The model under review builds one solid part; all positions refer to its coordinate system, in mm. A direction names the side the tool comes from. Coordinates: 2 decimals unless noted, no trailing zeros. Order: outer loops, then holes, each group sorted by start corner. A loop starts at its lowest first (then second) coordinate and runs counter-clockwise, first axis right, second up.
```python
from build123d import *

# Parameters (mm, degrees)
CROQUIS1_W              = 46
CROQUIS1_H              = 101
SALIENTE_EXTRUIR2_DEPTH = 4
CROQUIS2_R              = 2
CORTAR_EXTRUIR3_DEPTH   = 36
CROQUIS4_R              = 3
CORTAR_EXTRUIR4_DEPTH   = 2
REDONDEO1_R             = 5


with BuildPart() as part:
    # Croquis1 → Saliente-Extruir2 (new body)
    with BuildSketch(Plane(origin=(0, 0, 0), x_dir=(1, 0, 0), z_dir=(0, 1, 0))):
        Rectangle(CROQUIS1_W, CROQUIS1_H)
    extrude(amount=SALIENTE_EXTRUIR2_DEPTH)

    # Croquis2 → Cortar-Extruir3 (cut)
    with BuildSketch(Plane(origin=(0, 4, 0), x_dir=(1, 0, 0), z_dir=(0, 1, 0))):
        with Locations(Location((-15, 38.5, 0), (0, 0, 270))):
            Circle(CROQUIS2_R)
        with Locations(Location((15, 38.5, 0), (0, 0, 270))):
            Circle(CROQUIS2_R)
        with Locations(Location((-15, -38.5, 0), (0, 0, 270))):
            Circle(CROQUIS2_R)
        with Locations(Location((15, -38.5, 0), (0, 0, 270))):
            Circle(CROQUIS2_R)
    extrude(amount=-CORTAR_EXTRUIR3_DEPTH, mode=Mode.SUBTRACT)

    # Croquis4 → Cortar-Extruir4 (cut)
    with BuildSketch(Plane(origin=(0, 4, 0), x_dir=(1, 0, 0), z_dir=(0, 1, 0))):
        with Locations(Location((-15, -38.5, 0), (0, 0, 270))):
            Circle(CROQUIS4_R)
        with Locations(Location((15, -38.5, 0), (0, 0, 270))):
            Circle(CROQUIS4_R)
        with Locations(Location((-15, 38.5, 0), (0, 0, 270))):
            Circle(CROQUIS4_R)
        with Locations(Location((15, 38.5, 0), (0, 0, 270))):
            Circle(CROQUIS4_R)
    extrude(amount=-CORTAR_EXTRUIR4_DEPTH, mode=Mode.SUBTRACT)

    # Redondeo1
    redondeo1_edges = [part.edges().sort_by_distance(p)[0] for p in [
        (23, 2, 50.5),
        (-23, 2, 50.5),
        (-23, 2, -50.5),
        (23, 2, -50.5),
    ]]
    fillet(redondeo1_edges, radius=REDONDEO1_R)


solid = part.part
```
(1) Wall thickness on probe 1 along X at (y, z) = (1.2, -38.5); probe 2 along X at (y, z) = (3.55, -38.5); probe 3 along Z at (x, y) = (15.5, 1.4): over which ranges is each line inside the solid? List them lowest first.
A:
probe 1: x = -23 to -17, -13 to 13, 17 to 23
probe 2: x = -23 to -18, -12 to 12, 18 to 23
probe 3: z = -50.5 to -40.44, -36.56 to 36.56, 40.44 to 50.5
(2) Draft analysis for pull direction Z (two halves, no side actions). For faces 3 (the face through (0, 2, -50.5)), 4 (the face through (15, 2, 36)), 5 (the face through (0, 4, -1)), state which applies: released by +Z, released by -Z, zero draft, split by the parting line, or undercut.
A:
face 3: released by -Z
face 4: undercut
face 5: zero draft
(3) We need section B-B, the plane y = 0.8. Write out the cut boundary in (x, z), and give its area (3 significant figures).
A:
outline: (-23, -45.5) arc R5 ccw to (-18, -50.5) - (18, -50.5) arc R5 ccw to (23, -45.5) - (23, 45.5) arc R5 ccw to (18, 50.5) - (-18, 50.5) arc R5 ccw to (-23, 45.5) - close; hole circle Ø4 at (-15, -38.5); hole circle Ø4 at (-15, 38.5); hole circle Ø4 at (15, -38.5); hole circle Ø4 at (15, 38.5)
area: 4,570 mm2
(4) We need section C-C, the plane x = -15. Write out the cut boundary in (y, z), and give its area (3 significant figures).
A:
outline: (0, -50.5) - (4, -50.5) - (4, -41.5) - (2, -41.5) - (2, -40.5) - (0, -40.5) - close; (0, -36.5) - (2, -36.5) - (2, -35.5) - (4, -35.5) - (4, 35.5) - (2, 35.5) - (2, 36.5) - (0, 36.5) - close; (0, 40.5) - (2, 40.5) - (2, 41.5) - (4, 41.5) - (4, 50.5) - (0, 50.5) - close
area: 364 mm2
(5) We need section A-A, the plane z = 38.5. Write out the cut boundary in (x, y), and give its area (3 significant figures).
A:
outline: (-23, 0) - (-17, 0) - (-17, 2) - (-18, 2) - (-18, 4) - (-23, 4) - close; (-13, 0) - (13, 0) - (13, 2) - (12, 2) - (12, 4) - (-12, 4) - (-12, 2) - (-13, 2) - close; (17, 0) - (23, 0) - (23, 4) - (18, 4) - (18, 2) - (17, 2) - close
area: 144 mm2
(6) For pin 1 Ø3.5 at (x, z) = (-15, -38.5) entering from -Y; pin 2 Ø1.8 at (x, z) = (14, 37.5) entering from +Y, all flat-tipped, find the tip position at first contact; note any pin that passes through.
A:
pin 1: passes through
pin 2: stops at y = 2
(7) Machinability: for faces 1 (the face through (-15, 2, -41)), 2 (the face through (23, 2, 1)), which of the approach directions +Z, -Z, +X, -X, +Y, -Y give a long, thin tool a straight path to every point of the face, cutting with its end or side? Answer none if there is none.
A:
face 1: +Y
face 2: +Z, -Z, +X, +Y, -Y
